Input: part model. Units: mm. Frame: model coordinates. A direction names the side the tool comes from. Give positions to 0.01 mm unless a question says otherwise; leave off trailing zeros. Loops run counter-clockwise (first coordinate to the right, second up) from the corner with the lowest first, then second, coordinate; pieces in that order, holes last. Notation, with made-up numbers: (88.5, 11.25) - (117.5, 11.25) arc R19 ccw to (117.5, 16.25) - close; hole circle Ø9 at (69.5, 38.5). An arc over 180 degrees is marked (long way). One line per question, with ' | ' between items. Start each with the question number.
from build123d import *

# Parameters (mm, degrees)
SKETCH_1_W          = 130
SKETCH_1_H          = 30
SKETCH_1_R          = 1.45
EXTRUDE_1_DEPTH     = 5
SKETCH_3_W          = 16
SKETCH_3_H          = 3
CUT_EXTRUDE_1_DEPTH = 3
SKETCH_4_W          = 7
SKETCH_4_H          = 11
CUT_EXTRUDE_2_DEPTH = 67.895440801
SKETCH_6_W          = 34.5
SKETCH_6_H          = 25
SKETCH_6_W_2        = 10.5
SKETCH_6_H_2        = 9
SKETCH_6_W_3        = 9
SKETCH_6_H_3        = 5
CUT_EXTRUDE_3_DEPTH = 67.895440801
EXTRUDE_2_DEPTH     = 5
FILLET_1_R          = 2
FILLET_2_R          = 3
FILLET_3_R          = 1
FILLET_4_R          = 0.5


with BuildPart() as part:
    # 草图1 → 凸台-拉伸1 (new body)
    with BuildSketch(Plane.XY):
        Rectangle(SKETCH_1_W, SKETCH_1_H)
        with Locations((-57.5, -10)):
            Circle(SKETCH_1_R, mode=Mode.SUBTRACT)
        with Locations((-57.5, 10)):
            Circle(SKETCH_1_R, mode=Mode.SUBTRACT)
        with Locations(Location((57.5, -10, 0), (0, 0, 180))):
            Circle(SKETCH_1_R, mode=Mode.SUBTRACT)
        with Locations(Location((57.5, 10, 0), (0, 0, 180))):
            Circle(SKETCH_1_R, mode=Mode.SUBTRACT)
        with Locations((-15, 0)):
            Circle(SKETCH_1_R, mode=Mode.SUBTRACT)
        with Locations((15, 0)):
            Circle(SKETCH_1_R, mode=Mode.SUBTRACT)
    extrude(amount=EXTRUDE_1_DEPTH)

    # 草图3 → 切除-拉伸1 (cut)
    with BuildSketch(Plane.XY.offset(5)):
        Rectangle(SKETCH_3_W, SKETCH_3_H)
    extrude(amount=-CUT_EXTRUDE_1_DEPTH, mode=Mode.SUBTRACT)

    # 草图4 → 切除-拉伸2 (cut, through all)
    with BuildSketch(Plane.XY.offset(5)):
        Rectangle(SKETCH_4_W, SKETCH_4_H)
    extrude(amount=-CUT_EXTRUDE_2_DEPTH, mode=Mode.SUBTRACT)

    # 草图6 → 切除-拉伸3 (cut, through all)
    with BuildSketch(Plane.XY.offset(5)):
        Polygon((-65, 9.5), (-58, 5), (-58, -5), (-65, -9.5), align=None)
        with Locations((-37.25, 0)):
            Rectangle(SKETCH_6_W, SKETCH_6_H)
        with Locations((-11.75, 8.5)):
            Rectangle(SKETCH_6_W_2, SKETCH_6_H_2)
        with Locations((-11.75, -8.5)):
            Rectangle(SKETCH_6_W_2, SKETCH_6_H_2)
        with Locations((11.75, -8.5)):
            Rectangle(SKETCH_6_W_2, SKETCH_6_H_2)
        with Locations((11.75, 8.5)):
            Rectangle(SKETCH_6_W_2, SKETCH_6_H_2)
        with Locations((37.25, 0)):
            Rectangle(SKETCH_6_W, SKETCH_6_H)
        Polygon((65, -9.5), (65, 9.5), (58, 5), (58, -5), align=None)
        with Locations((0, 10)):
            Rectangle(SKETCH_6_W_3, SKETCH_6_H_3)
        with Locations((0, -10)):
            Rectangle(SKETCH_6_W_3, SKETCH_6_H_3)
    extrude(amount=-CUT_EXTRUDE_3_DEPTH, mode=Mode.SUBTRACT)

    # 草图7 → 凸台-拉伸2 (add)
    with BuildSketch(Plane.XY):
        Polygon((-54.5, 12.5), (-20, -10.108804199), (-20, -12.5), (-54.5, 10.108804199), align=None)
        Polygon((54.5, 12.5), (54.5, 10.108804199), (20, -12.5), (20, -10.108804199), align=None)
    extrude(amount=EXTRUDE_2_DEPTH)

    # 圆角1
    fillet_1_edges = [part.edges().sort_by_distance(p)[0] for p in [
        (-4.5, -12.5, 2.5),
        (-4.5, -7.5, 2.5),
        (4.5, -7.5, 2.5),
        (4.5, -12.5, 2.5),
        (6.5, -13, 2.5),
        (6.5, -4, 2.5),
        (17, -4, 2.5),
        (17, -13, 2.5),
        (-17, -4, 2.5),
        (-6.5, -4, 2.5),
        (-6.5, -13, 2.5),
        (-17, -13, 2.5),
        (-17, 13, 2.5),
        (-6.5, 13, 2.5),
        (-6.5, 4, 2.5),
        (-17, 4, 2.5),
        (-54.5, 12.5, 2.5),
        (-20, 12.5, 2.5),
        (-20, -12.5, 2.5),
        (-54.5, -12.5, 2.5),
        (-4.5, 7.5, 2.5),
        (-4.5, 12.5, 2.5),
        (4.5, 12.5, 2.5),
        (4.5, 7.5, 2.5),
        (20, -12.5, 2.5),
        (20, 12.5, 2.5),
        (54.5, 12.5, 2.5),
        (54.5, -12.5, 2.5),
        (6.5, 4, 2.5),
        (6.5, 13, 2.5),
        (17, 13, 2.5),
        (17, 4, 2.5),
        (-20, -10.108804199, 2.5),
        (-54.5, 10.108804199, 2.5),
        (54.5, 10.108804199, 2.5),
        (20, -10.108804199, 2.5),
    ]]
    fillet(fillet_1_edges, radius=FILLET_1_R)

    # 圆角2
    fillet_2_edges = [part.edges().sort_by_distance(p)[0] for p in [
        (-65, -9.5, 2.5),
        (-65, 9.5, 2.5),
        (-58, 5, 2.5),
        (-58, -5, 2.5),
        (65, -9.5, 2.5),
        (58, -5, 2.5),
        (58, 5, 2.5),
        (65, 9.5, 2.5),
        (65, -15, 2.5),
        (-65, -15, 2.5),
        (-65, 15, 2.5),
        (65, 15, 2.5),
    ]]
    fillet(fillet_2_edges, radius=FILLET_2_R)

    # 圆角3
    fillet_3_edges = [part.edges().sort_by_distance(p)[0] for p in [
        (3.5, 5.5, 2.5),
        (-3.5, -5.5, 2.5),
        (3.5, -5.5, 2.5),
        (-3.5, 5.5, 2.5),
    ]]
    fillet(fillet_3_edges, radius=FILLET_3_R)

    # 圆角4
    fillet_4_edges = [part.edges().sort_by_distance(p)[0] for p in [
        (8, 1.5, 3.5),
        (8, -1.5, 3.5),
        (-8, -1.5, 3.5),
        (-8, 1.5, 3.5),
    ]]
    fillet(fillet_4_edges, radius=FILLET_4_R)


solid = part.part
Q1. Access query for faces 4 (the face through (58.357, -4.781, 2.465)), 5 (the face through (5, -1.5, 4)), 6 (the face through (-64.643, -9.719, 2.465)), 7 (the face through (54.5, -2, 3)). Directions: +Z, -Z, +X, -X, +Y, -Y. A direction counts if a zero-diameter tool reaches every point of the face in a straight line with its end or side. Return the directions, or none.
Q2. Draft query along Y for faces 1 (the face through (-17, -9, 3)), 2 (the face through (-13.5, 3.5, 0)), 3 (the face through (0, -5.5, 3)). Return one class per face: +Y half, -Y half, draft (parallel to the pull), parting line (faces both ways), or undercut.
Q3. Line query: L1, parallel to Y at x = 15, z = 3.05; L2, parallel to Y at x = 57.5, z = 3.85; L3, parallel to Y at x = -13, z = 3. Output: solid intervals per line, ascending. Write a range as from..to.
Q4. First-contact query: pin 1 (1.5 mm diameter, centred on y = -8, z = 1.5, fed in from -X); pin 2 (3 mm diameter, centred on y = -2.5, z = 2.5, fed in from +X); pin 3 (0.8 mm diameter, centred on y = -10, z = 2.5, fed in from -X). Flat tips, straight axial feed; report the tip coordinate or a pass-through.
Q5. Section A-A, the plane x = -0.5. Output: boundary loops of the cut face in (y, z).
Q6. Section C-C, the plane z = 3.35. Count the separate pieces of the cut face and the enclosed holes in it, plus the area to 3 significant figures.
Q7. Section B-B, the plane x = 41. Output: boundary loops of the cut face in (y, z), plus the area to 3 significant figures.
Solved:
1) face 4: +Z, -Z, +X | face 5: +Z | face 6: +Z, -Z, -X | face 7: +Z, -Z
2) face 1: undercut | face 2: draft | face 3: undercut
3) L1: y = -15..-13, -4..-1.45, 1.45..4, 13..15 | L2: y = -15..-11.45, -8.55..8.55, 11.45..15 | L3: y = -15..-13, -4..4, 13..15
4) pin 1: stops at x = -63.82 | pin 2: stops at x = 58.07 | pin 3: stops at x = -64.91
5) outline: (-15, 0) - (-12.5, 0) - (-12.5, 5) - (-15, 5) - close; (-7.5, 0) - (-5.5, 0) - (-5.5, 5) - (-7.5, 5) - close; (5.5, 0) - (7.5, 0) - (7.5, 5) - (5.5, 5) - close; (12.5, 0) - (15, 0) - (15, 5) - (12.5, 5) - close
6) separate pieces: 1 | enclosed holes: 17 | area: 1,590 mm²
7) outline: (-15, 0) - (-12.5, 0) - (-12.5, 5) - (-15, 5) - close; (1.26, 0) - (3.65, 0) - (3.65, 5) - (1.26, 5) - close; (12.5, 0) - (15, 0) - (15, 5) - (12.5, 5) - close | area: 37.0 mm²
